Autodesk Inventor part; units mm, degrees
ref_plane "YZ Plane" through (0, 0, 0) normal (1, 0, 0) x (0, 1, 0)
ref_plane "XZ Plane" through (0, 0, 0) normal (0, 1, 0) x (-1, 0, 0)
ref_plane "XY Plane" through (0, 0, 0) normal (0, 0, 1) x (1, 0, 0)
sketch "草图1" plane through (0, 0, 0) normal (0, 0, 1) x (1, 0, 0)
  line L0 (0, 0) -> (72, 0)
  line L1 (72, 0) -> (72, -33)
  line L2 (72, -33) -> (0, -33)
  line L3 (0, -33) -> (0, 0)
  line L4 (36, 26.4753) -> (36, -41.1536) construction
  line L5 (0.9, -33) -> (71.1, -33) construction
  line L6 (71.1, -33) -> (71.1, 0) construction
  line L7 (71.1, 0) -> (0.9, 0) construction
  line L8 (0.9, 0) -> (0.9, -33) construction
  line L9 (0.9, -33) -> (71.1, 0) construction
  line L10 (71.1, -33) -> (0.9, 0) construction
  circle A0 centre (5.5, -18.9) radius 1 construction
  circle A1 centre (67.7, -18.9) radius 0.75
  circle A2 centre (5.5, -30.3) radius 0.75
  line L11 (0, -8) -> (-5, -8)
  line L12 (-5, -8) -> (-5, -28)
  line L13 (-5, -28) -> (0, -28)
  line L14 (0, -28) -> (0, -8)
  line L15 (72, -8) -> (77, -8)
  line L16 (77, -8) -> (77, -28)
  line L17 (77, -28) -> (72, -28)
  line L18 (72, -28) -> (72, -8)
  point P0 (36, -16.5)
  dimension "d0" = 72
  dimension "d1" = 70.2
  dimension "d2" = 33
  dimension "d3" = 0
  dimension "d4" = 0
  dimension "d5" = 2
  dimension "d6" = 18.9
  dimension "d7" = 4.6
  dimension "d8" = 1.5
  dimension "d9" = 62.2
  dimension "d10" = 1.5
  dimension "d11" = 11.4
  dimension "d12" = 5
  dimension "d13" = 20
  dimension "d14" = 5
  dimension "d15" = 5
  dimension "d16" = 20
  dimension "d17" = 5
extrude "拉伸1" add sketch "草图1" along normal blind 5
sketch "草图2" plane through (0, 0, 5) normal (0, 0, 1) x (1, 0, 0)
  circle A0 centre (67.7, -18.9) radius 0.75
  line L0 (0, -33) -> (72, -33)
  line L1 (72, -33) -> (72, -28)
  line L2 (-25.3854, -5.8) -> (85.4297, -5.8) construction
  line L3 (12.0239, -33) -> (63.7473, -33)
  line L4 (63.7473, -33) -> (63.7473, -28)
  line L5 (63.7473, -28) -> (12.0239, -28)
  line L6 (12.0239, -28) -> (12.0239, -33)
  dimension "d20" = 13.1
extrude "拉伸2" cut sketch "草图2" against normal through all contours L6 L5 L4 L0
properties part number "print-head-fix"
The model under review builds one solid part; all positions refer to its coordinate system, in mm. A direction names the side the tool comes from. Give positions to 0.01 mm unless a question says otherwise; leave off trailing zeros. Loops run counter-clockwise (first coordinate to the right, second up) from the corner with the lowest first, then second, coordinate; pieces in that order, holes last. Notation, with made-up numbers: (50, 79.25) -> (56, 79.25) arc R32 cw to (56, 106.25) -> close; hole circle Ø5 at (26, 84.25). An arc over 180 degrees is marked (long way). Answer as a JSON object with one key per item and string values. Group by question number.
Q1. Take a section at D-D (y = -4). Write out the cut boundary in (x, z).
Q2. Tool access review of faces 1 (the flat face through (74, -8, 2)), 2 (the flat face through (12.024, -30, 3)), 3 (the flat face through (75, -28, 2)), 4 (the flat face through (0, -31, 2)): name each direction out of +Z, -Z, +X, -X, +Y, -Y from which nothing blocks a thin tool from reaching the whole face with its end or side.
Q3. Insertion check: pin 1 (3 mm diameter, centred on x = 57.5, z = 4, fed in from +Y); pin 2 (1.5 mm diameter, centred on y = -31, z = 2.5, fed in from +X); pin 3 (2.5 mm diameter, centred on y = -4.5, z = 1.5, fed in from -X); pin 4 (1.5 mm diameter, centred on x = 45.5, z = 4, fed in from -Y). Each pin has a flat end and moves straight along its axis. Give the tip position at first contact, or say it passes through.
Q4. Take a section at A-A (y = -18.9). Write out the cut boundary in (x, z), plus the area to 4 significant figures.
Q5. Draft analysis for pull direction X (two halves, no side actions). For faces 5 (the flat face through (63.747, -31, 3)), 6 (the cylindrical face through (66.95, -18.93, 2.46)), 7 (the flat face through (72, -30, 2)), 8 (the flat face through (6, -33, 2)), state which applies: pulls with the +X half, pulls with the -X half, needs draft (parallel to the pull), parting line crosses it, or undercut.
Q6. Take a section at B-B (x = 67.7). Write out the cut boundary in (y, z), plus the area to 4 significant figures.
Q7. Take a section at C-C (z = 2.4). Write out the cut boundary in (x, y), plus the area to 3 significant figures.
Q8. Wall thickness on line 1 along Y through (x, z) = (5.5, 1.8); line 2 along X through (y, z) = (-19, 4.1); line 3 along Y through (x, z) = (18.5, 3.35): over which ranges is each line inside the solid? List them lowest first.
Answer below:
{
 "1": {"outline": "(0, 0) -> (72, 0) -> (72, 5) -> (0, 5) -> close"},
 "2": {"face 1": "+Z, -Z, +X, +Y", "face 2": "+Z, -Z, -Y", "face 3": "+Z, -Z, +X, -Y", "face 4": "+Z, -Z, -X, -Y"},
 "3": {"pin 1": "stops at y = 0", "pin 2": "stops at x = 72", "pin 3": "stops at x = 0", "pin 4": "stops at y = -28"},
 "4": {"outline": "(-5, 0) -> (66.95, 0) -> (66.95, 5) -> (-5, 5) -> close; (68.45, 0) -> (77, 0) -> (77, 5) -> (68.45, 5) -> close", "area": "402.5 mm2"},
 "5": {"face 5": "undercut", "face 6": "undercut", "face 7": "pulls with the +X half", "face 8": "needs draft"},
 "6": {"outline": "(-33, 0) -> (-19.65, 0) -> (-19.65, 5) -> (-33, 5) -> close; (-18.15, 0) -> (0, 0) -> (0, 5) -> (-18.15, 5) -> close", "area": "157.5 mm2"},
 "7": {"outline": "(-5, -28) -> (0, -28) -> (0, -33) -> (12.02, -33) -> (12.02, -28) -> (63.75, -28) -> (63.75, -33) -> (72, -33) -> (72, -28) -> (77, -28) -> (77, -8) -> (72, -8) -> (72, 0) -> (0, 0) -> (0, -8) -> (-5, -8) -> close; hole circle Ø1.5 at (5.5, -30.3); hole circle Ø1.5 at (67.7, -18.9)", "area": "2,310 mm2"},
 "8": {"line 1": "y = -33 to -31.05, -29.55 to 0", "line 2": "x = -5 to 66.96, 68.44 to 77", "line 3": "y = -28 to 0"}
}
